Could you check a few things on this model? Use its own coordinates, in mm. Face numbers are marked on the shaded views. A direction names the side the tool comes from. Coordinates: 2 decimals unless noted, no trailing zeros. Write each loop counter-clockwise with the first axis right and the second up, starting at its lowest first coordinate (ties: lowest second). Pieces come first, ordered by that corner, then holes. Notation, with made-up numbers: M 51,65 L 57,65 A29 ccw 57,96 Z; hole C 12.25,-16.75 d1. An arc over 180 degrees is marked long. Write item = value, one per line.
```python
from build123d import *

# Parameters (mm, degrees)
F2_DEPTH = 12.7
F3_DEPTH = 12.7


with BuildPart() as f2:
    # F0 (on Right) → F2 (new body)
    with BuildSketch(Plane.YZ):
        Polygon((-12.7, 31.75), (-12.7, 0), (12.7, 0), (12.7, 31.75), (6.35, 31.75), (6.35, 25.4), (-6.35, 25.4), (-6.35, 31.75), align=None)
    extrude(amount=F2_DEPTH)

    # F1 (on Right) → F3 (join)
    with BuildSketch(Plane.YZ):
        Polygon((-12.7, 31.75), (-12.7, 0), (12.7, 0), (12.7, 31.75), (6.35, 31.75), (6.35, 25.4), (-6.35, 25.4), (-6.35, 31.75), align=None)
    extrude(amount=-F3_DEPTH)


solid = f2.part
```
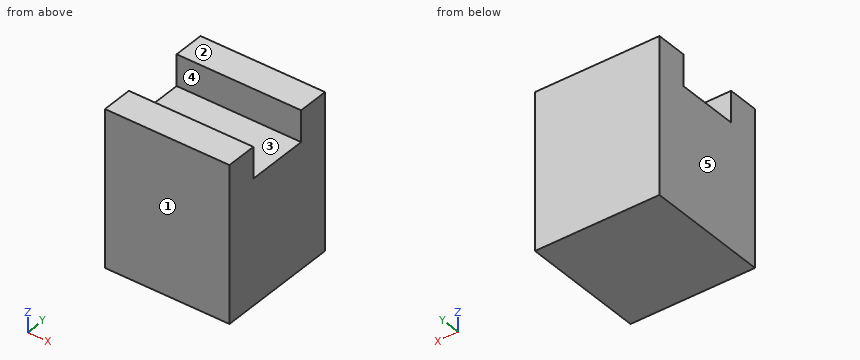
Item 1: I'm going to push a flat-ended pin straight in: P1, Ø6.5, axis at x = 4, y = -1, coming from the +Z side. Where does the tip first touch, or does it pass through?
Numbers:
P1 = 25.4
Item 2: If we mould it in two halves opening along Y, with no side actions, what happens to the marked faces 1, 2 and 3? For each: pulls with the +Y half, pulls with the -Y half, needs draft (parallel to the pull), parting line crosses it, or undercut.
Numbers:
face_1 = pulls with the -Y half
face_2 = needs draft
face_3 = undercut
Item 3: Imagine slicing it at B-B (y = -5.5). Write out the boundary of the cut face in (x, z).
Numbers:
outline = M -12.7,0 L 12.7,0 L 12.7,25.4 L -12.7,25.4 Z
Item 4: Imagine slicing it at A-A (x = 1.25). Write out the boundary of the cut face in (y, z).
Numbers:
outline = M -12.7,0 L 12.7,0 L 12.7,31.75 L 6.35,31.75 L 6.35,25.4 L -6.35,25.4 L -6.35,31.75 L -12.7,31.75 Z
Item 5: If I drill on line 1 along Y through (x, z) = (9.5, 25.5); line 2 along Z through (x, y) = (-11.5, -0.5), over which ranges is the centre line in solid material (lowest first)?
Numbers:
line_1 = -12.7 to -6.35, 6.35 to 12.7
line_2 = 0 to 25.4
Item 6: For the marked faces 4 and 5, which set-ups out of +Z, -Z, +X, -X, +Y, -Y let a thin tool reach every point of the face, with its end or its side?
Numbers:
face_4 = +Z, +X, -X
face_5 = +Z, -Z, -X, +Y, -Y
